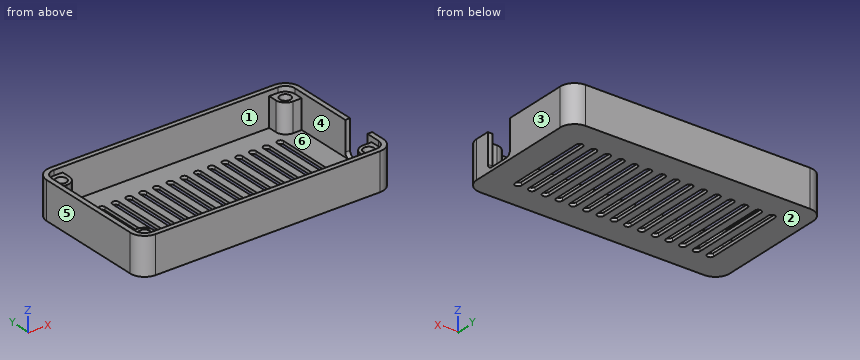
```python
from build123d import *

# Parameters (mm, degrees)
PAD_DEPTH           = 11.6
POCKET_DEPTH        = 10.6
PAD001_DEPTH        = 9
SKETCH003_R         = 1.7
POCKET001_DEPTH     = 6
POCKET002_DEPTH     = 5
POCKET003_DEPTH     = 5
LINEARPATTERN_COUNT = 15
LINEARPATTERN_PITCH = 4.285714


with BuildPart() as part:
    # Sketch → Pad (new body)
    with BuildSketch(Plane.XY):
        with BuildLine():
            Line((-35, 21.5), (35, 21.5))
            ThreePointArc((39.5, 17), (38.181981, 20.181981), (35, 21.5))
            Line((39.5, 17), (39.5, -17))
            ThreePointArc((35, -21.5), (38.181981, -20.181981), (39.5, -17))
            Line((35, -21.5), (-35, -21.5))
            ThreePointArc((-39.5, -17), (-38.181981, -20.181981), (-35, -21.5))
            Line((-39.5, -17), (-39.5, 17))
            ThreePointArc((-35, 21.5), (-38.181981, 20.181981), (-39.5, 17))
        make_face()
    extrude(amount=PAD_DEPTH)

    # Sketch001 (on Face10 of Pad) → Pocket (cut)
    with BuildSketch(Plane.XY.offset(11.6)):
        with BuildLine():
            Line((35, 20), (-35, 20))
            ThreePointArc((-35, 20), (-37.12132, 19.12132), (-38, 17))
            Line((-38, 17), (-38, -17))
            ThreePointArc((-38, -17), (-37.12132, -19.12132), (-35, -20))
            Line((-35, -20), (35, -20))
            ThreePointArc((35, -20), (37.12132, -19.12132), (38, -17))
            Line((38, -17), (38, 17))
            ThreePointArc((38, 17), (37.12132, 19.12132), (35, 20))
        make_face()
    extrude(amount=-POCKET_DEPTH, mode=Mode.SUBTRACT)

    # Sketch002 (on Face19 of Pocket) → Pad001 (join)
    with BuildSketch(Plane.XY.offset(1)):
        with BuildLine():
            Line((-35, 20), (-32.25, 20))
            Line((-32.25, 20), (-32.25, 17.25))
            ThreePointArc((-35.25, 14.25), (-33.12868, 15.12868), (-32.25, 17.25))
            Line((-35.25, 14.25), (-38, 14.25))
            Line((-38, 14.25), (-38, 17))
            ThreePointArc((-35, 20), (-37.12132, 19.12132), (-38, 17))
        make_face()
        with BuildLine():
            Line((35, 20), (32.25, 20))
            Line((32.25, 20), (32.25, 17.25))
            ThreePointArc((32.25, 17.25), (33.12868, 15.12868), (35.25, 14.25))
            Line((35.25, 14.25), (38, 14.25))
            Line((38, 14.25), (38, 17))
            ThreePointArc((38, 17), (37.12132, 19.12132), (35, 20))
        make_face()
        with BuildLine():
            Line((-38, -14.25), (-35.25, -14.25))
            ThreePointArc((-32.25, -17.25), (-33.12868, -15.12868), (-35.25, -14.25))
            Line((-32.25, -17.25), (-32.25, -20))
            Line((-32.25, -20), (-35, -20))
            ThreePointArc((-38, -17), (-37.12132, -19.12132), (-35, -20))
            Line((-38, -17), (-38, -14.25))
        make_face()
        with BuildLine():
            Line((35.25, -14.25), (38, -14.25))
            Line((38, -14.25), (38, -17))
            ThreePointArc((35, -20), (37.12132, -19.12132), (38, -17))
            Line((35, -20), (32.25, -20))
            Line((32.25, -20), (32.25, -17.25))
            ThreePointArc((35.25, -14.25), (33.12868, -15.12868), (32.25, -17.25))
        make_face()
    extrude(amount=PAD001_DEPTH)

    # Sketch003 (on Face19 of Pad001) → Pocket001 (cut)
    with BuildSketch(Plane.XY.offset(10)):
        with Locations((-35, 17)):
            Circle(SKETCH003_R)
        with Locations((-35, -17)):
            Circle(SKETCH003_R)
        with Locations((35, -17)):
            Circle(SKETCH003_R)
        with Locations((35, 17)):
            Circle(SKETCH003_R)
    extrude(amount=-POCKET001_DEPTH, mode=Mode.SUBTRACT)

    # Sketch009 (on Face9 of Pocket001) → Pocket002 (cut)
    with BuildSketch(Plane.YZ.offset(39.5)):
        with BuildLine():
            Line((-12.5, 11.6), (-3.5, 11.6))
            Line((-3.5, 11.6), (-3.5, 2.5))
            ThreePointArc((-5, 1), (-3.93934, 1.43934), (-3.5, 2.5))
            Line((-5, 1), (-11, 1))
            ThreePointArc((-12.5, 2.5), (-12.06066, 1.43934), (-11, 1))
            Line((-12.5, 2.5), (-12.5, 11.6))
        make_face()
    extrude(amount=-POCKET002_DEPTH, mode=Mode.SUBTRACT)

    # Sketch008 → Pocket003 (cut)
    with BuildSketch(Plane(origin=(0, 0, 0), x_dir=(1, 0, 0), z_dir=(0, 0, -1))):
        with BuildLine():
            ThreePointArc((-29, 12.5), (-30, 13.5), (-31, 12.5))
            Line((-31, 12.5), (-31, -12.5))
            ThreePointArc((-31, -12.5), (-30, -13.5), (-29, -12.5))
            Line((-29, -12.5), (-29, 12.5))
        make_face()
    pocket003 = extrude(amount=-POCKET003_DEPTH, mode=Mode.SUBTRACT)

    # LinearPattern: Pocket003 ×15
    with Locations(*[(i * LINEARPATTERN_PITCH, 0, 0) for i in range(1, LINEARPATTERN_COUNT)]):
        add(pocket003, mode=Mode.SUBTRACT)


solid = part.part
```
The listing builds one solid part. Answer for the finished solid, in the listing's coordinates (mm). Face numbers are marked on the shaded views. A direction names the side the tool comes from. Coordinates: 2 decimals unless noted, no trailing zeros. Write each loop counter-clockwise with the first axis right and the second up, starting at its lowest first coordinate (ties: lowest second). Pieces come first, ordered by that corner, then holes. Notation, with made-up numbers: (12.5, 40.25) -> (45.5, 40.25) arc R15 cw to (45.5, 58.25) -> close; hole circle Ø6 at (9.5, 52.5). An arc over 180 degrees is marked (long way). Write each question's results on one line, items separated by ' | '. Start each with the question number.
1) Flat-ended cylindrical pins translate along their axes: pin 1 Ø1.7 at (x, y) = (-34, -16) entering from +Z; pin 2 Ø2 at (x, y) = (35, 17) entering from +Z; pin 3 Ø3 at (x, y) = (19, -16) entering from +Z. Find the tip coordinate at first contact, or state that the pin passes through.
2) A cutting plane is placed at C-C (x = 19.5). Determine the outline of the cut face in (y, z).
3) A cutting plane is placed at B-B (x = -30). Determine the outline of the cut face in (y, z), then the cut area to 3 significant figures.
4) A tool of negligible diameter and unlimited length cuts with its end or side. For the marked faces 5 and 6, from which of +Z, -Z, +X, -X, +Y, -Y can it reach the whole face along a straight path? Write none if from no direction.
5) A cutting plane is placed at A-A (z = 9). Count the separate pieces of the cut face and the enclosed holes in it, then the cut area to 3 significant figures.
6) For a pull along X with two mould halves and no side action, classify the marked faces 1, 2, 3 and 4 as +X half, -X half, draft (parallel to the pull), parting line (faces both ways), or undercut.
7) Straight lines are drawn through the part: probe 1 along Y at (x, z) = (-35, 6.6); probe 2 along X at (y, z) = (5.5, 1.5); probe 3 along Y at (x, z) = (-24, 7.5). For each, find the intervals that lie inside material, in ascending order.
Values follow:
1) pin 1: z = 10 | pin 2: z = 4 | pin 3: z = 1
2) outline: (-21.5, 0) -> (21.5, 0) -> (21.5, 11.6) -> (20, 11.6) -> (20, 1) -> (-20, 1) -> (-20, 11.6) -> (-21.5, 11.6) -> close
3) outline: (-21.5, 0) -> (-13.5, 0) -> (-13.5, 1) -> (-20, 1) -> (-20, 11.6) -> (-21.5, 11.6) -> close; (13.5, 0) -> (21.5, 0) -> (21.5, 11.6) -> (20, 11.6) -> (20, 1) -> (13.5, 1) -> close | area: 47.8 mm²
4) face 5: +Z, -Z, -X, +Y, -Y | face 6: +Z
5) separate pieces: 1 | enclosed holes: 4 | area: 414 mm²
6) face 1: undercut | face 2: draft | face 3: +X half | face 4: undercut
7) probe 1: -21.5 to -18.7, -15.3 to -14.26, 14.26 to 15.3, 18.7 to 21.5 | probe 2: -39.5 to -38, 38 to 39.5 | probe 3: -21.5 to -20, 20 to 21.5
